Model file for the job. Use its own axes, mm. Face numbers are marked on the shaded views. A direction names the side the tool comes from. Give positions to 0.01 mm unless a question says otherwise; leave off trailing zeros. Loops run counter-clockwise (first coordinate to the right, second up) from the corner with the lowest first, then second, coordinate; pieces in that order, holes last. Notation, with made-up numbers: (46.5, 12.5) - (69.5, 12.5) arc R12 ccw to (69.5, 34.5) - close; hole circle Ø10 at (32, 22.25). An arc over 180 degrees is marked (long way). Use a Markdown table: item, result.
from build123d import *

# Parameters (mm, degrees)
BOSS_EXTRUDE5_DEPTH   = 10
CUT_EXTRUDE6_DEPTH    = 5
FILLET4_R             = 1
FILLET4_OF_MIRROR25_R = 1
BOSS_EXTRUDE6_DEPTH   = 4.9
MIRROR27_START        = 5.1
MIRROR27_DEPTH        = 4.9


# Read off the part's stored shape, not the designer's step: Mirror27
with BuildPart() as part:
    # Sketch15 → Boss-Extrude5 (new body)
    with BuildSketch(Plane(origin=(0, 0, 0), x_dir=(1, 0, 0), z_dir=(0, 1, 0))):
        Polygon((24.3, 76.900659127), (-6.625, 76.900659127), (-6.625, -4.5), (24.3, -4.5), (24.3, 44.900659127), (21.675, 44.900659127), (21.675, 47.400659127), (21.675, 72.400659127), (21.675, 74.900659127), (24.3, 74.900659127), align=None)
        Polygon((-2.625, 25), (-2.625, 0), (-2.625, -2.5), (0, -2.5), (2.625, -2.5), (2.625, 0), (2.625, 25), (2.625, 27.5), (0, 27.5), (-2.625, 27.5), align=None, mode=Mode.SUBTRACT)
    boss_extrude5 = extrude(amount=BOSS_EXTRUDE5_DEPTH)

    # Sketch18 → Cut-Extrude6 (cut)
    with BuildSketch(Plane(origin=(0, 10, 0), x_dir=(1, 0, 0), z_dir=(0, 1, 0))):
        Polygon((21.675, 51.3980649), (-4.44053483, 51.3980649), (-4.44053483, 20.8980649), (24.3, 20.8980649), (24.3, 51.3980649), align=None)
    cut_extrude6 = extrude(amount=-CUT_EXTRUDE6_DEPTH, mode=Mode.SUBTRACT)

    # Fillet4
    fillet4_edges = [part.edges().sort_by_distance(p)[0] for p in [
        (21.675, 5, -74.900659127),
        (-2.625, 5, 2.5),
        (2.625, 5, 2.5),
        (2.625, 2.5, -27.5),
        (-2.625, 2.5, -27.5),
        (21.675, 2.5, -44.900659127),
    ]]
    fillet(fillet4_edges, radius=FILLET4_R)

    # Mirror25: Boss-Extrude5, Cut-Extrude6 across plane
    add(boss_extrude5.mirror(Plane(origin=(24.3, 10, 4.5), x_dir=(0, 0, 1), z_dir=(-1, 0, 0))))
    add(cut_extrude6.mirror(Plane(origin=(24.3, 10, 4.5), x_dir=(0, 0, 1), z_dir=(-1, 0, 0))), mode=Mode.SUBTRACT)

    # Fillet4 of Mirror25
    fillet4_of_mirror25_edges = [part.edges().sort_by_distance(p)[0] for p in [
        (26.925, 5, -74.900659127),
        (51.225, 5, 2.5),
        (45.975, 5, 2.5),
        (45.975, 2.5, -27.5),
        (51.225, 2.5, -27.5),
        (26.925, 2.5, -44.900659127),
    ]]
    fillet(fillet4_of_mirror25_edges, radius=FILLET4_OF_MIRROR25_R)


with BuildPart() as body_2:
    # Sketch19 → Boss-Extrude6 (new body)
    with BuildSketch(Plane(origin=(0, 10, 0), x_dir=(1, 0, 0), z_dir=(0, 1, 0))):
        with BuildLine():
            Line((2.625, 21.1480649), (2.625, 26.5))
            ThreePointArc((2.625, 26.5), (2.332106781, 27.207106781), (1.625, 27.5))
            Line((1.625, 27.5), (-1.625, 27.5))
            ThreePointArc((-1.625, 27.5), (-2.332106781, 27.207106781), (-2.625, 26.5))
            Line((-2.625, 26.5), (-2.625, 21.1480649))
            Line((-2.625, 21.1480649), (-4.34053483, 21.1480649))
            Line((-4.34053483, 21.1480649), (-4.34053483, 41.1480649))
            Line((-4.34053483, 41.1480649), (24.3, 41.1480649))
            Line((24.3, 41.1480649), (24.3, 33.7730649))
            Line((24.3, 33.7730649), (0.65946517, 33.7730649))
            ThreePointArc((0.65946517, 33.7730649), (-1.96553483, 31.1480649), (0.65946517, 28.5230649))
            Line((0.65946517, 28.5230649), (24.3, 28.5230649))
            Line((24.3, 28.5230649), (24.3, 21.1480649))
            Line((24.3, 21.1480649), (2.625, 21.1480649))
        make_face()
    extrude(amount=-BOSS_EXTRUDE6_DEPTH)

    # Mirror27 outline → Mirror27 (add)
    with BuildSketch(Plane(origin=(0, 0, 0), x_dir=(1, 0, 0), z_dir=(0, 1, 0)).offset(MIRROR27_START)):
        with BuildLine():
            ThreePointArc((45.975, 26.5), (46.267893219, 27.207106781), (46.975, 27.5))
            Line((46.975, 27.5), (50.225, 27.5))
            ThreePointArc((50.225, 27.5), (50.932106781, 27.207106781), (51.225, 26.5))
            Line((51.225, 26.5), (51.225, 21.1480649))
            Line((51.225, 21.1480649), (52.94053483, 21.1480649))
            Line((52.94053483, 21.1480649), (52.94053483, 41.1480649))
            Line((52.94053483, 41.1480649), (24.3, 41.1480649))
            Line((24.3, 41.1480649), (24.3, 33.7730649))
            Line((24.3, 33.7730649), (47.94053483, 33.7730649))
            ThreePointArc((47.94053483, 33.7730649), (50.56553483, 31.1480649), (47.94053483, 28.5230649))
            Line((47.94053483, 28.5230649), (24.3, 28.5230649))
            Line((24.3, 28.5230649), (24.3, 21.1480649))
            Line((24.3, 21.1480649), (45.975, 21.1480649))
            Line((45.975, 21.1480649), (45.975, 26.5))
        make_face()
    extrude(amount=MIRROR27_DEPTH)


solid = body_2.part
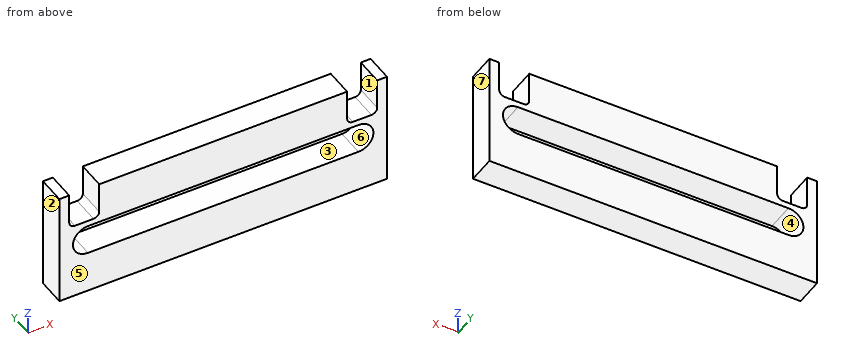
(1) Slice it at D-D, the plane z = -32. Write the cut outline in (x, y), plus the area to 3 significant figures.
Computed:
| item | result |
|---|---|
| outline | (-4.34, 5.1) - (-1.82, 5.1) - (-1.82, 10) - (-4.34, 10) - close; (50.42, 5.1) - (52.94, 5.1) - (52.94, 10) - (50.42, 10) - close |
| area | 24.7 mm² |
(2) Slice it at B-B, the plane z = -23. Write the cut outline in (x, y) (3 decimals).
Computed:
| item | result |
|---|---|
| outline | (-4.341, 5.1) - (-2.625, 5.1) - (-2.625, 10) - (-4.341, 10) - close; (2.625, 5.1) - (45.975, 5.1) - (45.975, 10) - (2.625, 10) - close; (51.225, 5.1) - (52.941, 5.1) - (52.941, 10) - (51.225, 10) - close |
(3) Mould opens along X. For the marked faces 4, 5, 6 and 7 say: pulls with the +X half, pulls with the -X half, needs draft (parallel to the pull), parting line crosses it, or undercut.
Computed:
| item | result |
|---|---|
| face 4 | undercut |
| face 5 | needs draft |
| face 6 | undercut |
| face 7 | pulls with the +X half |
(4) Slice it at C-C, the plane y = 9.25. Write the cut outline in (x, z) (3 decimals), plus the area to 3 significant figures.
Computed:
| item | result |
|---|---|
| outline | (-4.341, -41.148) - (52.941, -41.148) - (52.941, -21.148) - (51.225, -21.148) - (51.225, -26.5) arc R1 cw to (50.225, -27.5) - (46.975, -27.5) arc R1 cw to (45.975, -26.5) - (45.975, -21.148) - (2.625, -21.148) - (2.625, -26.5) arc R1 cw to (1.625, -27.5) - (-1.625, -27.5) arc R1 cw to (-2.625, -26.5) - (-2.625, -21.148) - (-4.341, -21.148) - close; hole (0.659, -33.773) - (47.941, -33.773) arc R2.625 ccw to (47.941, -28.523) - (0.659, -28.523) arc R2.625 ccw to start |
| area | 810 mm² |
(5) 3-axis set-ups, long thin cutter, end or side, ignore diameter. For the marked faces 1, 2 and 3: which of +Z, -Z, +X, -X, +Y, -Y reach the whole face in a straight line?
Computed:
| item | result |
|---|---|
| face 1 | +Z, +Y, -Y |
| face 2 | +Z, -Z, -X, +Y, -Y |
| face 3 | +Y, -Y |
(6) Pin check, flat tips, straight feed: P1, Ø2.5, axis at x = 0.5, y = 7, coming from the +Z side; P2, Ø8, axis at x = 2.5, z = -25.5, coming from the -Y side. Stop position of each tip, or through.
Computed:
| item | result |
|---|---|
| P1 | z = -27.49 |
| P2 | y = 5.1 |
(7) Slice it at A-A, the plane x = 26.5. Write the cut outline in (y, z).
Computed:
| item | result |
|---|---|
| outline | (5.1, -41.15) - (10, -41.15) - (10, -33.77) - (5.1, -33.77) - close; (5.1, -28.52) - (10, -28.52) - (10, -21.15) - (5.1, -21.15) - close |
(8) Drill centre lines: probe 1 along X at (y, z) = (8.25, -22.5) (3 decimals); probe 2 along Z at (x, y) = (29.5, 6.3); probe 3 along Z at (x, y) = (47, 7.25). Where is each one in solid material? Low to high. Write a range as [from, to].
Computed:
| item | result |
|---|---|
| probe 1 | [-4.341, -2.625], [2.625, 45.975], [51.225, 52.941] |
| probe 2 | [-41.15, -33.77], [-28.52, -21.15] |
| probe 3 | [-41.15, -33.77], [-28.52, -27.5] |
